from build123d import *

# Parameters (mm, degrees)
EXTRUDE1_DEPTH     = 45.65
FILLET1_R          = 1
SKETCH2_R          = 1.15
CUT_EXTRUDE1_DEPTH = 1
SKETCH3_R          = 2.84
SKETCH3_R_2        = 2
EXTRUDE2_DEPTH     = 2.54
FILLET2_R          = 0.4
SKETCH4_W          = 3.5
SKETCH4_H          = 1.4
EXTRUDE3_DEPTH     = 2.54
CUT_EXTRUDE2_DEPTH = 4
CUT_EXTRUDE3_DEPTH = 4
CIRPATTERN2_COUNT  = 6


with BuildPart() as part:
    # Sketch1 → Extrude1 (new body)
    with BuildSketch(Plane(origin=(0, 0, 0), x_dir=(1, 0, 0), z_dir=(0, 1, 0))):
        with BuildLine():
            Line((-9.25, 8.55), (9.25, 8.55))
            ThreePointArc((9.25, 8.55), (12.078427125, 7.378427125), (13.25, 4.55))
            Line((13.25, 4.55), (13.25, -4.55))
            ThreePointArc((13.25, -4.55), (12.078427125, -7.378427125), (9.25, -8.55))
            Line((9.25, -8.55), (-9.25, -8.55))
            ThreePointArc((-9.25, -8.55), (-12.078427125, -7.378427125), (-13.25, -4.55))
            Line((-13.25, -4.55), (-13.25, 4.55))
            ThreePointArc((-13.25, 4.55), (-12.078427125, 7.378427125), (-9.25, 8.55))
        make_face()
    extrude(amount=EXTRUDE1_DEPTH)

    # Fillet1
    fillet1_edges = [part.edges().sort_by_distance(p)[0] for p in [
        (-12.078427125, 45.65, -7.378427125),
        (-13.25, 45.65, 0),
        (-12.078427125, 45.65, 7.378427125),
        (0, 45.65, 8.55),
        (12.078427125, 45.65, 7.378427125),
        (13.25, 45.65, 0),
        (12.078427125, 45.65, -7.378427125),
        (13.25, 0, 0),
        (0, 45.65, -8.55),
        (12.078427125, 0, 7.378427125),
        (0, 0, 8.55),
        (-12.078427125, 0, 7.378427125),
        (-13.25, 0, 0),
        (-12.078427125, 0, -7.378427125),
        (0, 0, -8.55),
        (12.078427125, 0, -7.378427125),
    ]]
    fillet(fillet1_edges, radius=FILLET1_R)

    # Sketch2 → Cut-Extrude1 (cut)
    with BuildSketch(Plane(origin=(0, 45.65, 0), x_dir=(-1, 0, 0), z_dir=(0, 1, 0))):
        with Locations(Location((6.35, 0, 0), (0, 0, 90))):  # turned: the seam where the file's is
            Circle(SKETCH2_R)
        with Locations(Location((-6.35, 0, 0), (0, 0, 90))):  # turned: the seam where the file's is
            Circle(SKETCH2_R)
    extrude(amount=-CUT_EXTRUDE1_DEPTH, mode=Mode.SUBTRACT)

    # Sketch3 → Extrude2 (add)
    with BuildSketch(Plane(origin=(0, 45.65, 0), x_dir=(-1, 0, 0), z_dir=(0, 1, 0))):
        with Locations(Location((6.35, 0, 0), (0, 0, 270))):  # turned: the seam where the file's is
            Circle(SKETCH3_R)
        with Locations(Location((6.35, 0, 0), (0, 0, 90))):  # turned: the seam where the file's is
            Circle(SKETCH3_R_2, mode=Mode.SUBTRACT)
    extrude(amount=EXTRUDE2_DEPTH)

    # Fillet2
    fillet2_edges = [part.edges().sort_by_distance(p)[0] for p in [
        (-6.35, 48.19, 2.84),
        (-6.35, 48.19, -2),
    ]]
    fillet(fillet2_edges, radius=FILLET2_R)

    # Sketch4 → Extrude3 (add)
    with BuildSketch(Plane(origin=(0, 45.65, 0), x_dir=(-1, 0, 0), z_dir=(0, 1, 0))):
        with Locations((-6.35, -3.5)):
            Rectangle(SKETCH4_W, SKETCH4_H)
    extrude3 = extrude(amount=EXTRUDE3_DEPTH)

    # Sketch5 → Cut-Extrude2 (cut)
    with BuildSketch(Plane(origin=(8.1, 0, 0), x_dir=(0, 0, -1), z_dir=(1, 0, 0))):
        with BuildLine():
            Line((4.13400445, 45.65), (4.55, 45.65))
            Line((4.55, 45.65), (4.55, 48.403159162))
            Line((4.55, 48.403159162), (2.544765199, 48.403159162))
            Line((2.544765199, 48.403159162), (2.544765199, 45.65))
            Line((2.544765199, 45.65), (3.5, 45.65))
            ThreePointArc((3.5, 45.65), (3.535730788, 46.560835661), (3.754944335, 47.445620218))
            ThreePointArc((3.754944335, 47.445620218), (3.65385849, 47.619389121), (3.5, 47.49))
            ThreePointArc((3.5, 47.49), (3.15, 47.14), (2.8, 47.49))
            ThreePointArc((2.8, 47.49), (3.620027609, 48.179632781), (4.158838209, 47.253500074))
            ThreePointArc((4.158838209, 47.253500074), (4.013267709, 46.453812217), (4.13400445, 45.65))
        make_face()
    cut_extrude2 = extrude(amount=-CUT_EXTRUDE2_DEPTH, mode=Mode.SUBTRACT)

    # Sketch6 → Cut-Extrude3 (cut)
    with BuildSketch(Plane(origin=(0, 45.65, 0), x_dir=(-1, 0, 0), z_dir=(0, 1, 0))):
        Polygon((-7.781645023, -2.8), (-8.1, -2.8), (-8.1, -3.115078907), align=None)
        Polygon((-4.6, -2.8), (-4.918354977, -2.8), (-4.6, -3.115078907), align=None)
    cut_extrude3 = extrude(amount=CUT_EXTRUDE3_DEPTH, mode=Mode.SUBTRACT)

    # CirPattern2: Extrude3, Cut-Extrude2, Cut-Extrude3 ×6 about axis
    cirpattern2_axis = Axis((6.35, 0, 0), (0, 1, 0))
    add([extrude3.rotate(cirpattern2_axis, i * 360 / CIRPATTERN2_COUNT) for i in range(1, CIRPATTERN2_COUNT)])
    add([cut_extrude2.rotate(cirpattern2_axis, i * 360 / CIRPATTERN2_COUNT) for i in range(1, CIRPATTERN2_COUNT)], mode=Mode.SUBTRACT)
    add([cut_extrude3.rotate(cirpattern2_axis, i * 360 / CIRPATTERN2_COUNT) for i in range(1, CIRPATTERN2_COUNT)], mode=Mode.SUBTRACT)


solid = part.part
CAD build for the part. Positions are in the model's coordinates, mm. A direction names the side the tool comes from. Round coordinates to 2 decimals unless told otherwise and drop trailing zeros. Write each loop counter-clockwise with the first axis right and the second up, starting at its lowest first coordinate (ties: lowest second). Pieces come first, ordered by that corner, then holes.
(1) Drop flat-ended pins along their axis: P1, Ø1.8, axis at x = -6, z = 0, coming from the +Y side; P2, Ø0.9, axis at y = 47, z = -3.5, coming from the -X side; P3, Ø1.2, axis at y = 46.5, z = 4, coming from the -X side. Give the stop position or say it passes through.
(2) Slice it at C-C, the plane x = 6.35. Write the cut outline in (y, z).
(3) Probe line 1 along Y through (x, z) = (1.75, 6); line 2 along X through (y, z) = (2, -7.5); line 3 along X through (y, z) = (38.5, 7). List the from-to ranges inside material, lowest first.
(4) Slice it at B-B, the plane x = -0.75. Write the cut outline in (y, z).
(5) Slice it at A-A, the plane y = 43. Write the cut outline in (x, z), and give its area (3 significant figures).
(6) Mould opens along Z. For faces 4 (the face through (0.13, 0.301, -8.265)), 5 (the face through (6.325, 46.465, 4.013)), 6 (the face through (6.374, 48.182, -3.603)) say: pulls with the +Z half, pulls with the -Z half, needs draft (parallel to the pull), parting line crosses it, or undercut.
(7) 3-axis set-ups, long thin cutter, end or side, ignore diameter. For faces 1 (the face through (8.753, 46.902, -3.408)), 2 (the face through (3.947, 46.902, 3.408)), 3 (the face through (6, 44.65, 0)): which of +Z, -Z, +X, -X, +Y, -Y reach the whole face in a straight line?
From the geometry:
1. P1: stops at y = 45.65
1. P2: stops at x = 3.35
1. P3: stops at x = 3.68
2. outline: (0, -7.55) arc R1 ccw to (1, -8.55) - (44.65, -8.55) arc R1 ccw to (45.65, -7.55) - (45.65, -4.13) arc R2.48 cw to (47.25, -4.16) arc R0.7 ccw (long way) to (47.49, -2.8) arc R0.35 ccw to (47.49, -3.5) arc R0.13 cw (long way) to (47.45, -3.75) arc R4.48 ccw to (45.65, -3.5) - (45.65, -1.15) - (44.65, -1.15) - (44.65, 1.15) - (45.65, 1.15) - (45.65, 3.5) arc R4.48 ccw to (47.45, 3.75) arc R0.13 cw (long way) to (47.49, 3.5) arc R0.35 ccw to (47.49, 2.8) arc R0.7 ccw (long way) to (47.25, 4.16) arc R2.48 cw to (45.65, 4.13) - (45.65, 7.55) arc R1 ccw to (44.65, 8.55) - (1, 8.55) arc R1 ccw to (0, 7.55) - close
3. line 1: y = 0 to 45.65
3. line 2: x = -11.95 to 11.95
3. line 3: x = -12.41 to 12.41
4. outline: (0, -7.55) arc R1 ccw to (1, -8.55) - (44.65, -8.55) arc R1 ccw to (45.65, -7.55) - (45.65, 7.55) arc R1 ccw to (44.65, 8.55) - (1, 8.55) arc R1 ccw to (0, 7.55) - close
5. outline: (-13.25, -4.55) arc R4 ccw to (-9.25, -8.55) - (9.25, -8.55) arc R4 ccw to (13.25, -4.55) - (13.25, 4.55) arc R4 ccw to (9.25, 8.55) - (-9.25, 8.55) arc R4 ccw to (-13.25, 4.55) - close
5. area: 439 mm2
6. face 4: pulls with the -Z half
6. face 5: pulls with the +Z half
6. face 6: undercut
7. face 1: -Z, +Y
7. face 2: +Z, +Y
7. face 3: +Y
